from build123d import *

# Parameters (mm, degrees)
SKETCH1_R           = 1.5
BOSS_EXTRUDE1_DEPTH = 4
SKETCH2_R           = 2.25
BOSS_EXTRUDE2_DEPTH = 4
FILLET1_R           = 8
FILLET2_R           = 5


with BuildPart() as part:
    # Sketch1 → Boss-Extrude1 (new body)
    with BuildSketch(Plane(origin=(0, 0, 0), x_dir=(1, 0, 0), z_dir=(0, 1, 0))):
        with BuildLine():
            Line((10, 140), (10, 0))
            Line((10, 0), (0, 0))
            Line((0, 0), (0, 140))
            ThreePointArc((0, 140), (5, 145), (10, 140))
        make_face()
        with Locations((5, 120)):
            Circle(SKETCH1_R, mode=Mode.SUBTRACT)
    extrude(amount=BOSS_EXTRUDE1_DEPTH)

    # Sketch2 → Boss-Extrude2 (add)
    with BuildSketch(Plane(origin=(0, 4, 0), x_dir=(1, 0, 0), z_dir=(0, 1, 0))):
        with BuildLine():
            Line((70, 0), (10, 0))
            Line((10, 0), (0, 0))
            Line((0, 0), (0, -10))
            Line((0, -10), (70, -10))
            ThreePointArc((70, -10), (75, -5), (70, 0))
        make_face()
        with Locations((5, -5)):
            Circle(SKETCH2_R, mode=Mode.SUBTRACT)
        with Locations((19, -5)):
            Circle(SKETCH2_R, mode=Mode.SUBTRACT)
        with Locations((56, -5)):
            Circle(SKETCH2_R, mode=Mode.SUBTRACT)
        with Locations((70, -5)):
            Circle(SKETCH2_R, mode=Mode.SUBTRACT)
    extrude(amount=-BOSS_EXTRUDE2_DEPTH)

    # Fillet1
    fillet1_edges = [part.edges().sort_by_distance(p)[0] for p in [
        (10, 2, 0),
    ]]
    fillet(fillet1_edges, radius=FILLET1_R)

    # Fillet2
    fillet2_edges = [part.edges().sort_by_distance(p)[0] for p in [
        (0, 2, 10),
    ]]
    fillet(fillet2_edges, radius=FILLET2_R)


solid = part.part
For this review, take the finished solid that the model builds, in its own axes (mm). A direction names the side the tool comes from. Round coordinates to 2 decimals unless told otherwise and drop trailing zeros. Write each loop counter-clockwise with the first axis right and the second up, starting at its lowest first coordinate (ties: lowest second). Pieces come first, ordered by that corner, then holes. Notation, with made-up numbers: M 88,8.5 L 122,8.5 A21 cw 122,20.5 Z; hole C 7,30 d1. An arc over 180 degrees is marked long. Write item = value, one per line. Start each with the question number.
(1) We need section A-A (x = 56). Give the boundary of the cut face in (y, z).
(2) For faces 1 (the face through (37, 2, 10)), 2 (the face through (44, 2, 0)), list the 3-axis set-ups (+Z, -Z, +X, -X, +Y, -Y) from which the entire face can be reached by the end or side of a thin tool; tool diameter is ignored.
(3) Clearance check with flat-ended pins moving along their axes: pin 1 Ø3.5 at (x, z) = (5, 5) entering from +Y; pin 2 Ø5 at (x, z) = (56, 5) entering from +Y. State where each tip first meets the part, or that it passes through.
(4) The part is to be moulded in two halves that separate along X. For faces 3 (the face through (53.752, 2.028, 4.901)), 4 (the face through (9.5, 4, -44.9)), 5 (the face through (10, 2, -75)), say which applies: +X half, -X half, draft (parallel to the pull), parting line (faces both ways), or undercut.
(5) For line 1 along Z through (x, y) = (5, 2.3); line 2 along Z through (x, y) = (70, 2.8); line 3 along X through (y, z) = (1.9, -120), list the stretches that pass through material, from the lowest coordinate up.
(6) We need section B-B (z = -120). Give the boundary of the cut face in (x, y), then the cut area to 3 significant figures.
(7) We need section C-C (y = 1.15). Give the boundary of the cut face in (x, z).
(8) We need section D-D (z = -78). Give the boundary of the cut face in (x, y), then the cut area to 3 significant figures.
Results found:
q1.outline = M 0,0 L 4,0 L 4,2.75 L 0,2.75 Z; M 0,7.25 L 4,7.25 L 4,10 L 0,10 Z
q2.face_1 = +Z, +X, -X, +Y, -Y
q2.face_2 = -Z, +X, +Y, -Y
q3.pin_1 = through
q3.pin_2 = 4
q4.face_3 = undercut
q4.face_4 = draft
q4.face_5 = +X half
q5.line_1 = -145 to -121.5, -118.5 to 2.75, 7.25 to 10
q5.line_2 = 0 to 2.75, 7.25 to 10
q5.line_3 = 0 to 3.5, 6.5 to 10
q6.outline = M 0,0 L 3.5,0 L 3.5,4 L 0,4 Z; M 6.5,0 L 10,0 L 10,4 L 6.5,4 Z
q6.area = 28.0 mm²
q7.outline = M 0,-140 A5 ccw 10,-140 L 10,-8 A8 cw 18,0 L 70,0 A5 ccw 70,10 L 5,10 A5 ccw 0,5 Z; hole C 5,5 d4.5; hole C 5,-120 d3; hole C 19,5 d4.5; hole C 56,5 d4.5; hole C 70,5 d4.5
q8.outline = M 0,0 L 10,0 L 10,4 L 0,4 Z
q8.area = 40.0 mm²
